from build123d import *

# Parameters (mm, degrees)
SKETCH1_R           = 39.5
BOSS_EXTRUDE1_DEPTH = 40
CUT_EXTRUDE2_DEPTH  = 41
CUT_EXTRUDE3_DEPTH  = 41
FILLET2_R           = 1
SKETCH6_W           = 114.3
SKETCH6_H           = 9
BOSS_EXTRUDE2_DEPTH = 40
FILLET6_R           = 10
CUT_EXTRUDE4_REACH  = 42
SKETCH9_R           = 3.3782
SKETCH11_W          = 31.75
SKETCH11_H          = 9
BOSS_EXTRUDE3_DEPTH = 29.21
SKETCH4_W           = 3.002871012
SKETCH4_H           = 30
FILLET7_R           = 3.302
SKETCH13_R          = 5.08
CUT_EXTRUDE6_DEPTH  = 5.08
SKETCH15_R          = 3.3782
CUT_EXTRUDE8_DEPTH  = 10
SKETCH16_R          = 5.08
CUT_EXTRUDE9_DEPTH  = 5.08
SKETCH17_W          = 36.586278343
SKETCH17_H          = 70.835632368
CUT_EXTRUDE10_DEPTH = 10
FILLET8_R           = 3.302


with BuildPart() as part:
    # Sketch1 → Boss-Extrude1 (new body)
    with BuildSketch(Plane.XY):
        Circle(SKETCH1_R)
    extrude(amount=BOSS_EXTRUDE1_DEPTH)

    # Sketch2 → Cut-Extrude2 (cut, through all)
    with BuildSketch(Plane(origin=(0, 0, 0), x_dir=(-1, 0, 0), z_dir=(0, 0, -1))):
        with BuildLine():
            Line((-39.5, 0), (39.5, 0))
            ThreePointArc((39.5, 0), (0, -39.5), (-39.5, 0))
        make_face()
    extrude(amount=-CUT_EXTRUDE2_DEPTH, mode=Mode.SUBTRACT)

    # Sketch3 → Cut-Extrude3 (cut, through all)
    with BuildSketch(Plane(origin=(0, 0, 0), x_dir=(-1, 0, 0), z_dir=(0, 0, -1))):
        with BuildLine():
            Line((-29.5, 0), (29.5, 0))
            ThreePointArc((29.5, 0), (0, 29.5), (-29.5, 0))
        make_face()
    extrude(amount=-CUT_EXTRUDE3_DEPTH, mode=Mode.SUBTRACT)

    # Fillet2
    fillet2_edges = [part.edges().sort_by_distance(p)[0] for p in [
        (-34.5, 0, 0),
        (-34.5, 0, 40),
        (0, 29.5, 40),
        (29.5, 0, 20),
        (-29.5, 0, 20),
        (0, 29.5, 0),
        (-39.5, 0, 20),
        (34.5, 0, 0),
        (39.5, 0, 20),
        (34.5, 0, 40),
    ]]
    fillet(fillet2_edges, radius=FILLET2_R)

    # Sketch6 → Boss-Extrude2 (add)
    with BuildSketch(Plane(origin=(0, 0, 0), x_dir=(-1, 0, 0), z_dir=(0, 0, -1))):
        with Locations((0, 35.5)):
            Rectangle(SKETCH6_W, SKETCH6_H)
    extrude(amount=-BOSS_EXTRUDE2_DEPTH)

    # Fillet6
    fillet6_edges = [part.edges().sort_by_distance(p)[0] for p in [
        (-24.47958333, 31, 20),
        (24.47958333, 31, 20),
    ]]
    fillet(fillet6_edges, radius=FILLET6_R)

    # Sketch9 → Cut-Extrude4 (cut, up to next)
    with BuildSketch(Plane(origin=(0, 40, 0), x_dir=(1, 0, 0), z_dir=(0, 1, 0)), mode=Mode.PRIVATE) as cut_extrude4_sk1:
        with Locations((-50.677371465, -7.173)):
            Circle(SKETCH9_R)
    cut_extrude4_tool1 = extrude(cut_extrude4_sk1.sketch, amount=-CUT_EXTRUDE4_REACH, mode=Mode.PRIVATE) & part.part
    add(cut_extrude4_tool1.solids().sort_by_distance((-50.677371, 40, 7.173))[0], mode=Mode.SUBTRACT)
    # Sketch9 → Cut-Extrude4 (cut, up to next)
    with BuildSketch(Plane(origin=(0, 40, 0), x_dir=(1, 0, 0), z_dir=(0, 1, 0)), mode=Mode.PRIVATE) as cut_extrude4_sk2:
        with Locations((-50.677371465, -32.827)):
            Circle(SKETCH9_R)
    cut_extrude4_tool2 = extrude(cut_extrude4_sk2.sketch, amount=-CUT_EXTRUDE4_REACH, mode=Mode.PRIVATE) & part.part
    add(cut_extrude4_tool2.solids().sort_by_distance((-50.677371, 40, 32.827))[0], mode=Mode.SUBTRACT)

    # Sketch11 → Boss-Extrude3 (add)
    with BuildSketch(Plane.XY.offset(40)):
        with Locations((41.275, 35.5)):
            Rectangle(SKETCH11_W, SKETCH11_H)
    extrude(amount=BOSS_EXTRUDE3_DEPTH)

    # Sketch4 → Cut-Revolve1 (revolve, cut)
    with BuildSketch(Plane.XZ):
        with Locations((34.48557529, 20)):
            Rectangle(SKETCH4_W, SKETCH4_H)
    revolve(axis=Axis((0, 0, 0), (0, 0, 1)), mode=Mode.SUBTRACT)

    # Fillet7
    fillet7_edges = [part.edges().sort_by_distance(p)[0] for p in [
        (25.4, 35.5, 40),
        (25.4, 35.5, 69.21),
        (57.15, 35.5, 69.21),
        (-57.15, 35.5, 0),
        (57.15, 35.5, 0),
        (-57.15, 35.5, 40),
    ]]
    fillet(fillet7_edges, radius=FILLET7_R)

    # Sketch13 → Cut-Extrude6 (cut)
    with BuildSketch(Plane.XZ.offset(-31)):
        with Locations((-50.677371465, 32.827)):
            Circle(SKETCH13_R)
        with Locations((-50.677371465, 7.173)):
            Circle(SKETCH13_R)
    extrude(amount=-CUT_EXTRUDE6_DEPTH, mode=Mode.SUBTRACT)

    # Sketch15 → Cut-Extrude8 (cut, through all)
    with BuildSketch(Plane.XZ.offset(-31)):
        with Locations((31.75, 62.86)):
            Circle(SKETCH15_R)
    extrude(amount=-CUT_EXTRUDE8_DEPTH, mode=Mode.SUBTRACT)

    # Sketch16 → Cut-Extrude9 (cut)
    with BuildSketch(Plane.XZ.offset(-31)):
        with Locations((31.75, 62.86)):
            Circle(SKETCH16_R)
    extrude(amount=-CUT_EXTRUDE9_DEPTH, mode=Mode.SUBTRACT)

    # Sketch17 → Cut-Extrude10 (cut, through all)
    with BuildSketch(Plane.XZ.offset(-31)):
        with Locations((63.117797564, 35.417816184)):
            Rectangle(SKETCH17_W, SKETCH17_H)
    extrude(amount=-CUT_EXTRUDE10_DEPTH, mode=Mode.SUBTRACT)

    # Fillet8
    fillet8_edges = [part.edges().sort_by_distance(p)[0] for p in [
        (44.824658392, 35.5, 69.21),
        (44.824658392, 35.5, 0),
    ]]
    fillet(fillet8_edges, radius=FILLET8_R)


with BuildPart() as body_2:
    # Mirror8: mirrored copy
    add(part.part.mirror(Plane(origin=(-57.15, 40, 154.653783191), x_dir=(0, 0, 1), z_dir=(-1, 0, 0))))


solid = part.part
Design review of the part built by this model. Coordinates are the model's own, in mm. A direction names the side the tool comes from. Give positions to 0.01 mm unless a question says otherwise; leave off trailing zeros. Order: outer loops, then holes, each group sorted by start corner. A loop starts at its lowest first (then second) coordinate and runs counter-clockwise, first axis right, second up.
1. Add section B-B, the plane x = 0. State the section outline as (y, z) points.
Solution:
outline: (29.5, 1) arc R1 ccw to (30.5, 0) - (40, 0) - (40, 40) - (30.5, 40) arc R1 ccw to (29.5, 39) - close; hole (32.98, 5) - (35.99, 5) - (35.99, 35) - (32.98, 35) - close
2. Add section A-A, the plane z = 62.86. State the section outline as (x, y) points, then the cut area to 3 significant figures.
Solution:
outline: (25.4, 31) - (26.67, 31) - (26.67, 36.08) - (28.37, 36.08) - (28.37, 40) - (25.4, 40) - close; (35.13, 36.08) - (36.83, 36.08) - (36.83, 31) - (44.82, 31) - (44.82, 40) - (35.13, 40) - close
area: 96.7 mm2
3. Mouldability with a two-part tool opening along Y and no side actions: class faces 4 (the cylindrical face through (0.79, 35.98, 20.21)), 5 (the cylindrical face through (-0.635, 29.493, 19.734)), 6 (the cylindrical face through (-56.157, 35.563, 0.942)) as +Y half, -Y half, draft (parallel to the pull), parting line (faces both ways), or undercut.
Solution:
face 4: undercut
face 5: -Y half
face 6: draft
4. Add section C-C, the plane x = 31.75. State the section outline as (y, z) points.
Solution:
outline: (0, 1) arc R1 ccw to (1, 0) - (40, 0) - (40, 59.48) - (36.08, 59.48) - (36.08, 57.78) - (31, 57.78) - (31, 40) - (1, 40) arc R1 ccw to (0, 39) - close; (31, 67.94) - (36.08, 67.94) - (36.08, 66.24) - (40, 66.24) - (40, 69.21) - (31, 69.21) - close; hole (8.94, 5) - (16.94, 5) - (16.94, 35) - (8.94, 35) - close
5. To check wall thickness, follow L1, parallel to X at y = 3.5, z = 30.5; L2, parallel to X at y = 33.5, z = 63; L3, parallel to Z at x = -22, y = 25.5. State the ranges of each line that lie inside material, in increasing order.
Solution:
L1: x = -39.34 to -35.82, -32.8 to -29.29, 29.29 to 32.8, 35.82 to 39.34
L2: x = 25.4 to 26.67, 36.83 to 44.82
L3: z = 0 to 5, 35 to 40
6. Tool access review of faces 1 (the flat face through (25.4, 35, 54)), 2 (the cylindrical face through (-45.985, 33.504, 5.227)), 3 (the flat face through (-15, 29, 40)): name each direction out of +Z, -Z, +X, -X, +Y, -Y from which nothing blocks a thin tool from reaching the whole face with its end or side.
Solution:
face 1: +Z, -X, +Y, -Y
face 2: -Y
face 3: +Z, -X, -Y
7. Add section D-D, the plane y = 12. State how many separate pieces and enclosed holes the cut face has, then the cut area to 3 significant figures.
Solution:
separate pieces: 2
enclosed holes: 2
area: 662 mm2
8. For pin 1 Ø1.5 at (y, z) = (8, 12.5) entering from +X; pin 2 Ø3 at (x, z) = (30.5, 61) entering from -Y; pin 3 Ø2 at (y, z) = (26, 40) entering from +X, all flat-tipped, find the tip position at first contact; note any pin that passes through.
Solution:
pin 1: stops at x = 38.83
pin 2: stops at y = 36.08
pin 3: stops at x = 36.82
